Part model, mm, in its own coordinate system. A direction names the side the tool comes from. Round coordinates to 2 decimals unless told otherwise and drop trailing zeros. Write each loop counter-clockwise with the first axis right and the second up, starting at its lowest first coordinate (ties: lowest second). Pieces come first, ordered by that corner, then holes. Notation, with made-up numbers: M 26,-3 L 39,-3 A24 ccw 39,27 Z; hole C 85.5,-20 d7. An arc over 180 degrees is marked long. Use a Markdown table: item, result. Add a question column.
1) Two-plate mould, pull along X, no slides. Class faces 1 (the face through (-1, 17.5, -11)), 2 (the face through (-1, 55, -2)), 3 (the face through (-40.5, 29, -1)): released by +X, released by -X, zero draft, split by the parting line, or undercut.
2) Slice it at B-B on y = 52. Write the cut outline in (x, z) (3 decimals), plus the area to 4 significant figures.
3) Slice it at A-A on y = 38. Write the cut outline in (x, z) (3 decimals), plus the area to 4 significant figures.
4) Slice it at C-C on z = 2.5. Give the number of separate pieces and of enclosed holes in the cut face, plus the area to 4 significant figures.
5) Which spindle directions (+Z, -Z, +X, -X, +Y, -Y) get a long thin tool onto all of the face, cutting with end or side? Do faces 4 (the face through (-1, 56, -1)), 5 (the face through (-46, 1, 4.75)), 6 (the face through (-1, 41, -11)). Say none if no direction does.
6) Wall check: probe 1 along X at (y, z) = (24, -7) (3 decimals); probe 2 along X at (y, z) = (54, 4.5); probe 3 along Z at (x, y) = (8, 14.5). Give the ranges that are in metal, low to high.
7) Drop flat-ended pins along their axis: P1, Ø6, axis at y = 18, z = -2, coming from the +X side; P2, Ø8, axis at x = -8, y = 31.5, coming from the +Z side; P3, Ø0.5, axis at x = -40, z = 3, coming from the -Y side; P4, Ø0.5, axis at x = 40, y = 28, coming from the -Z side. Give the stop position or say it passes through.
```python
from build123d import *

# Parameters (mm, degrees)
BOSS_EXTRUDE1_DEPTH = 2
BOSS_EXTRUDE4_DEPTH = 95.75
SKETCH3_W           = 81
SKETCH3_H           = 19.5
BOSS_EXTRUDE5_DEPTH = 54
SKETCH4_W           = 10
SKETCH4_H           = 2.5
CUT_EXTRUDE1_DEPTH  = 1
SHELL1_START        = -39.5
SHELL1_OUTLINE_W    = 54
SHELL1_OUTLINE_H    = 19.5
SHELL1_DEPTH        = 79
SKETCH4_2_W         = 10
SKETCH4_2_H         = 2.5
CUT_EXTRUDE2_DEPTH  = 106.789664547
CUT_EXTRUDE3_REACH  = 107.79
SKETCH5_W           = 10
SKETCH5_H           = 18.5
SKETCH6_W           = 66
SKETCH6_H           = 11
CUT_EXTRUDE4_DEPTH  = 1


# Read off the part's stored shape, not the designer's step: Shell1
with BuildPart() as part:
    # Sketch1 → Boss-Extrude1 (new body)
    with BuildSketch(Plane(origin=(0, 0, 0), x_dir=(1, 0, 0), z_dir=(0, 1, 0))):
        with BuildLine():
            Line((-47.875, -4.75), (-47.875, -13.75))
            Line((-47.875, -13.75), (47.875, -13.75))
            Line((47.875, -13.75), (47.875, -4.75))
            Line((47.875, -4.75), (43.375, -4.75))
            ThreePointArc((43.375, -4.75), (41.125, -2.5), (43.375, -0.25))
            Line((43.375, -0.25), (47.875, -0.25))
            Line((47.875, -0.25), (47.875, 13.75))
            Line((47.875, 13.75), (-47.875, 13.75))
            Line((-47.875, 13.75), (-47.875, -0.25))
            Line((-47.875, -0.25), (-43.375, -0.25))
            ThreePointArc((-43.375, -0.25), (-41.125, -2.5), (-43.375, -4.75))
            Line((-43.375, -4.75), (-47.875, -4.75))
        make_face()
    extrude(amount=BOSS_EXTRUDE1_DEPTH)

    # Sketch2 → Boss-Extrude4 (add)
    with BuildSketch(Plane.ZY.offset(47.875)):
        Polygon((-13.75, 0), (-6.25, 0), (-6.25, 56.5), (-13.75, 56.5), (-13.75, 54.5), (-8.25, 54.5), (-8.25, 47.5), (-13.75, 47.5), (-13.75, 47), (-8.25, 47), (-8.25, 41.5), (-13.75, 41.5), (-13.75, 41), (-8.25, 41), (-8.25, 35.5), (-13.75, 35.5), (-13.75, 35), (-8.25, 35), (-8.25, 29.5), (-13.75, 29.5), (-13.75, 29), (-8.25, 29), (-8.25, 23.5), (-13.75, 23.5), (-13.75, 23), (-8.25, 23), (-8.25, 17.5), (-13.75, 17.5), (-13.75, 17), (-8.25, 17), (-8.25, 2), (-13.75, 2), align=None)
    extrude(amount=-BOSS_EXTRUDE4_DEPTH)

    # Sketch3 → Boss-Extrude5 (add)
    with BuildSketch(Plane(origin=(0, 2, 0), x_dir=(1, 0, 0), z_dir=(0, 1, 0))):
        with Locations((0, -3.5)):
            Rectangle(SKETCH3_W, SKETCH3_H)
    extrude(amount=BOSS_EXTRUDE5_DEPTH)

    # Sketch4 → Cut-Extrude1 (cut)
    with BuildSketch(Plane(origin=(40.5, 0, 0), x_dir=(0, 0, -1), z_dir=(1, 0, 0))):
        with Locations((-3.5, 47.75)):
            Rectangle(SKETCH4_W, SKETCH4_H)
        with Locations((-3.5, 42.75)):
            Rectangle(SKETCH4_W, SKETCH4_H)
        with Locations((-3.5, 37.75)):
            Rectangle(SKETCH4_W, SKETCH4_H)
        with Locations((-3.5, 32.75)):
            Rectangle(SKETCH4_W, SKETCH4_H)
        with Locations((-3.5, 27.75)):
            Rectangle(SKETCH4_W, SKETCH4_H)
        with Locations((-3.5, 22.75)):
            Rectangle(SKETCH4_W, SKETCH4_H)
        with Locations((-3.5, 17.75)):
            Rectangle(SKETCH4_W, SKETCH4_H)
        with Locations((-3.5, 12.75)):
            Rectangle(SKETCH4_W, SKETCH4_H)
    extrude(amount=-CUT_EXTRUDE1_DEPTH, mode=Mode.SUBTRACT)

    # Shell1 outline → Shell1 (cut)
    with BuildSketch(Plane.YZ.offset(SHELL1_START)):
        with Locations((28, 2.5)):
            Rectangle(SHELL1_OUTLINE_W, SHELL1_OUTLINE_H)
    extrude(amount=SHELL1_DEPTH, mode=Mode.SUBTRACT)

    # Sketch4<2> → Cut-Extrude2 (cut, through all)
    with BuildSketch(Plane(origin=(40.5, 0, 0), x_dir=(0, 0, -1), z_dir=(1, 0, 0))):
        with Locations((-3.5, 47.75)):
            Rectangle(SKETCH4_2_W, SKETCH4_2_H)
        with Locations((-3.5, 17.75)):
            Rectangle(SKETCH4_2_W, SKETCH4_2_H)
        with Locations((-3.5, 12.75)):
            Rectangle(SKETCH4_2_W, SKETCH4_2_H)
    extrude(amount=-CUT_EXTRUDE2_DEPTH, mode=Mode.SUBTRACT)

    # Sketch5 → Cut-Extrude3 (cut, up to next)
    with BuildSketch(Plane.ZY.offset(40.5), mode=Mode.PRIVATE) as cut_extrude3_sk1:
        with Locations((5, 30.25)):
            Rectangle(SKETCH5_W, SKETCH5_H)
    cut_extrude3_tool1 = extrude(cut_extrude3_sk1.sketch, amount=-CUT_EXTRUDE3_REACH, mode=Mode.PRIVATE) & part.part
    add(cut_extrude3_tool1.solids().sort_by_distance((-40.5, 30.25, 5))[0], mode=Mode.SUBTRACT)

    # Sketch6 → Cut-Extrude4 (cut)
    with BuildSketch(Plane(origin=(0, 56, 0), x_dir=(1, 0, 0), z_dir=(0, 1, 0))):
        with Locations((0, -4.75)):
            Rectangle(SKETCH6_W, SKETCH6_H)
    extrude(amount=-CUT_EXTRUDE4_DEPTH, mode=Mode.SUBTRACT)


solid = part.part
```
Entries:
| question | item | result |
|---|---|---|
| 1 | face 1 | zero draft |
| 1 | face 2 | undercut |
| 1 | face 3 | released by -X |
| 2 | outline | M -47.875,-8.25 L 47.875,-8.25 L 47.875,-6.25 L 40.5,-6.25 L 40.5,13.25 L -40.5,13.25 L -40.5,-6.25 L -47.875,-6.25 Z; hole M -39.5,-7.25 L 39.5,-7.25 L 39.5,12.25 L -39.5,12.25 Z |
| 2 | area | 230.5 mm^2 |
| 3 | outline | M -47.875,-8.25 L 47.875,-8.25 L 47.875,-6.25 L 40.5,-6.25 L 40.5,-1.5 L 39.5,-1.5 L 39.5,-7.25 L -39.5,-7.25 L -39.5,0 L -40.5,0 L -40.5,-6.25 L -47.875,-6.25 Z; M -40.5,10 L -39.5,10 L -39.5,12.25 L 39.5,12.25 L 39.5,8.5 L 40.5,8.5 L 40.5,13.25 L -40.5,13.25 Z |
| 3 | area | 210.5 mm^2 |
| 4 | separate pieces | 13 |
| 4 | enclosed holes | 0 |
| 4 | area | 160.5 mm^2 |
| 5 | face 4 | +Z, +X, -X, +Y |
| 5 | face 5 | -X, +Y, -Y |
| 5 | face 6 | -Z, +X, -X |
| 6 | probe 1 | x = -47.875 to -39.5, 39.5 to 47.875 |
| 6 | probe 2 | x = -40.5 to -39.5, 39.5 to 40.5 |
| 6 | probe 3 | z = -8.25 to -7.25, 12.25 to 13.25 |
| 7 | P1 | stops at x = 40.5 |
| 7 | P2 | stops at z = 13.25 |
| 7 | P3 | stops at y = 0 |
| 7 | P4 | stops at z = -8.25 |
